from build123d import *

# Parameters (mm, degrees)
F3_SIZE = 0.5
F4_SIZE = 0.5


with BuildPart() as f2:
    # F1 (on Front) → F2 (revolve)
    with BuildSketch(Plane.XZ):
        Polygon((-16.05, 0), (-13.05, 0), (-13.05, 45.823673), (-14.05, 46), (-14.05, 55), (-24.05, 55), (-24.05, 54), (-16.05, 51.856406), align=None)
        Polygon((-24.05, -55), (-14.05, -55), (-14.05, -46), (-13.05, -45.823673), (-13.05, 0), (-16.05, 0), (-16.05, -51.856406), (-24.05, -54), align=None)
    revolve(axis=Axis((0, 0, 37.963357), (0, 0, 1)))

    # F3
    f3_edges = [f2.edges().sort_by_distance(p)[0] for p in [
        (14.05, 0, -55),
        (14.05, 0, 55),
        (24.05, 0, -55),
        (24.05, 0, 55),
    ]]
    chamfer(f3_edges, length=F3_SIZE)

    # F4
    f4_edges = [f2.edges().sort_by_distance(p)[0] for p in [
        (13.05, 0, 45.823673),
        (13.05, 0, -45.823673),
    ]]
    chamfer(f4_edges, length=F4_SIZE)


solid = f2.part
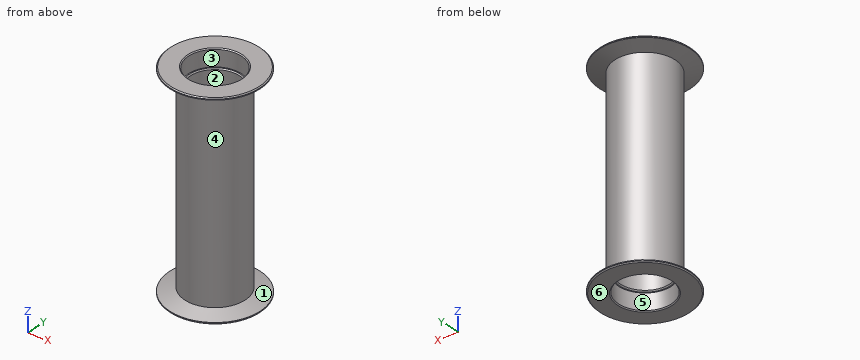
Verification items for the finished model (mm, model axes). Face numbers are marked on the shaded views. A direction names the side the tool comes from. Coordinates: 2 decimals unless noted, no trailing zeros. Order: outer loops, then holes, each group sorted by start corner. A loop starts at its lowest first (then second) coordinate and runs counter-clockwise, first axis right, second up. Notation, with made-up numbers: (25, -3.5) -> (54, -3.5) arc R15 ccw to (54, 16.5) -> close; hole circle Ø10 at (23, -14). An arc over 180 degrees is marked (long way). Put each result on its own line as item: value. Start each with the question number.
1. Mould release check, pull along Y, two halves, no side actions. Record for the marked faces 4, 5 and 6: released by +Y, released by -Y, zero draft, split by the parting line, or undercut.
2. Access from +Z, -Z, +X, -X, +Y, -Y to the whole of each face (thin tool, end or side, straight path). Record for the marked faces 1, 2 and 3.
3. Go/stop test with flat-tipped pins: pin 1 Ø1.5 at (x, z) = (-11, -0.5) entering from +Y; pin 2 Ø6 at (y, z) = (4, 3.5) entering from +X; pin 3 Ø5 at (y, z) = (-13, -32.5) entering from +X. Record where each tip stops, or that it passes through.
4. Material ranges on L1, parallel to Y at x = 0, z = -50; L2, parallel to X at y = -0.5, z = 20, recorded low to high. Write a range as [from, to].
5. Cross-section at A-A, the plane z = 31. Record the boundary of the cut face in (x, y).
Computed:
1. face 4: split by the parting line
1. face 5: undercut
1. face 6: zero draft
2. face 1: none
2. face 2: +Z, -Z
2. face 3: +Z
3. pin 1: y = 12.35
3. pin 2: x = 16.02
3. pin 3: x = 12.14
4. L1: [-16.05, -14.05], [14.05, 16.05]
4. L2: [-16.04, -13.04], [13.04, 16.04]
5. outline: circle Ø32.1 at (0, 0); hole circle Ø26.1 at (0, 0)
